Geometry check sheet. Reference: drawing and pictorial views, mm from the part's lowest x, y, z. Give positions to 0.01 mm unless a question says otherwise; leave off trailing zeros. Order: outer loops, then holes, each group sorted by start corner. A loop starts at its lowest first (then second) coordinate and runs counter-clockwise, first axis right, second up.
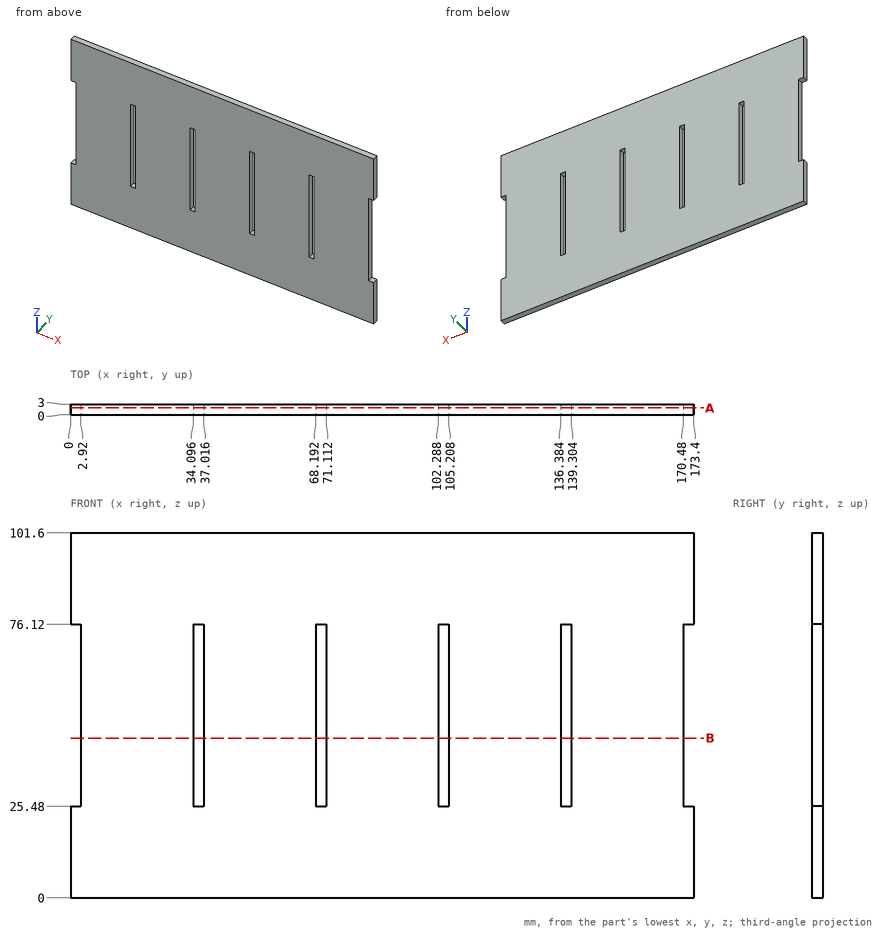
(1) Cross-section at A-A on y = 1.95. Enter the section's corners in (x, z).
Response values:
outline: (0, 0) - (173.4, 0) - (173.4, 25.48) - (170.48, 25.48) - (170.48, 76.12) - (173.4, 76.12) - (173.4, 101.6) - (0, 101.6) - (0, 76.12) - (2.92, 76.12) - (2.92, 25.48) - (0, 25.48) - close; hole (34.1, 25.48) - (37.02, 25.48) - (37.02, 76.12) - (34.1, 76.12) - close; hole (68.19, 25.48) - (71.11, 25.48) - (71.11, 76.12) - (68.19, 76.12) - close; hole (102.29, 25.48) - (105.21, 25.48) - (105.21, 76.12) - (102.29, 76.12) - close; hole (136.38, 25.48) - (139.3, 25.48) - (139.3, 76.12) - (136.38, 76.12) - close
(2) Cross-section at B-B on z = 44.5. Enter the section's corners in (x, y), then the cut area to 3 significant figures.
Response values:
outline: (2.92, 0) - (34.1, 0) - (34.1, 3) - (2.92, 3) - close; (37.02, 0) - (68.19, 0) - (68.19, 3) - (37.02, 3) - close; (71.11, 0) - (102.29, 0) - (102.29, 3) - (71.11, 3) - close; (105.21, 0) - (136.38, 0) - (136.38, 3) - (105.21, 3) - close; (139.3, 0) - (170.48, 0) - (170.48, 3) - (139.3, 3) - close
area: 468 mm2
(3) Gauge pin test, flat ends, axial feed: pin 1 Ø1.5 at (y, z) = (1.5, 39.5) entering from -X; pin 2 Ø0.9 at (y, z) = (2, 48) entering from +X; pin 3 Ø0.9 at (x, y) = (1.5, 2) entering from -Z. Record the tip position at first contact, or that the pin passes through.
Response values:
pin 1: stops at x = 2.92
pin 2: stops at x = 170.48
pin 3: stops at z = 0
(4) Material ranges on L1, parallel to X at y = 2.3, z = 71; L2, parallel to Z at x = 102.5, y = 2.5, recorded low to high.
Response values:
L1: x = 2.92 to 34.1, 37.02 to 68.19, 71.11 to 102.29, 105.21 to 136.38, 139.3 to 170.48
L2: z = 0 to 25.48, 76.12 to 101.6
